Check sheet for the modelled part. Datum: model origin and axes. Units: mm. Coordinates: 2 decimals unless noted, no trailing zeros. Loops run counter-clockwise (first coordinate to the right, second up) from the corner with the lowest first, then second, coordinate; pieces in that order, holes last. Notation, with made-up numbers: (-0.75, -13) - (17.25, -13) arc R13 cw to (17.25, 10) - close; hole circle Ø5 at (-7, 82). An arc over 180 degrees is marked (long way). Use a Markdown table: item, result. Add a question column.
1) Thickness scan on line 1 (X direction, y = 1.8, z = -20); line 2 (Z direction, x = 20, y = 2.65); line 3 (Z direction, x = 29, y = 1.2). Record the ranges inside material, lowest first.
2) Draft check along Z on faces 1 (the cylindrical face through (16.29, 2.465, -17.635)), 2 (the flat face through (0, 2, -51)), 3 (the flat face through (20, 2, 0)), 4 (the flat face through (20, 2, -100)). Enter one of: pulls with the +Z half, pulls with the -Z half, needs draft (parallel to the pull), parting line crosses it, or undercut.
3) Sectioned sample at C-C, the plane x = 20. Enter the section's corners in (y, z), then the cut area to 3 significant figures.
4) Sectioned sample at B-B, the plane z = -20. Enter the section's corners in (x, y).
5) Sectioned sample at D-D, the plane y = 3.55. Enter the section's corners in (x, z), then the cut area to 3 significant figures.
6) Sectioned sample at A-A, the plane x = 36. Enter the section's corners in (y, z).
7) Go/stop test with a flat-tipped pin: P1, Ø1, axis at y = 2.5, z = -11.5, coming from the -X side. Record where the tip stops, or that it passes through.
Autodesk Inventor part; units mm, degrees
ref_plane "YZ Plane" through (0, 0, 0) normal (1, 0, 0) x (0, 1, 0)
ref_plane "XZ Plane" through (0, 0, 0) normal (0, 1, 0) x (-1, 0, 0)
ref_plane "XY Plane" through (0, 0, 0) normal (0, 0, 1) x (1, 0, 0)
sketch "スケッチ1" plane through (0, 0, 0) normal (0, 1, 0) x (-1, 0, 0)
  line L0 (0, 0) -> (-40, 0)
  line L1 (-40, 0) -> (-40, -100)
  line L2 (-40, -100) -> (0, -100)
  line L3 (0, -100) -> (0, 0)
  dimension "d0" = 40
  dimension "d1" = 100
extrude "押し出し1" add sketch "スケッチ1" along normal blind 5
sketch "スケッチ2" plane through (0, 5, 0) normal (0, 1, 0) x (1, 0, 0)
  line L0 (0, 0) -> (40, 0) construction
  line L1 (20, 0) -> (20, 100) construction
  line L2 (40, 100) -> (0, 100) construction
  point P0 (20, 20)
  dimension "d4" = 20
hole "穴1" at (20, 5, -20) direction (0, -1, 0) diameter 8.8 end through all
sketch "スケッチ3" plane through (0, 5, 0) normal (0, 1, 0) x (1, 0, 0)
  circle A0 centre (20, 20) radius 4.4 construction
  circle A1 centre (20, 20) radius 9 construction
  point P0 (0, 0)
  point P1 (11, 20)
  point P2 (20, 11)
  point P3 (29, 20)
  point P4 (20, 29)
  dimension "d12" = 18
  dimension "d15" = 360
hole "穴2" at (11, 5, -20) at (20, 5, -11) at (29, 5, -20) at (20, 5, -29) direction (0, -1, 0) diameter 4.4 end through all
sketch "スケッチ4" plane through (0, 5, 0) normal (0, 1, 0) x (1, 0, 0)
  line L0 (40, 100) -> (0, 100) construction
  line L1 (0, 100) -> (40, 100) construction
  line L2 (40, 100) -> (40, 95) construction
  line L3 (40, 95) -> (0, 95) construction
  line L4 (0, 95) -> (0, 100) construction
  line L5 (0, 100) -> (0, 0)
  line L6 (0, 97.5) -> (40, 97.5) construction
  line L7 (40, 0) -> (40, 100)
  point P0 (4, 97.5)
  point P1 (36, 97.5)
  dimension "d25" = 5
  dimension "d26" = 4
  dimension "d27" = 4
hole "穴3" at (4, 5, -97.5) at (36, 5, -97.5) direction (0, -1, 0) diameter 2.459 end through all
properties part number "shoulder1_sidel_plate"
Solved:
| question | item | result |
|---|---|---|
| 1 | line 1 | x = 0 to 8.8, 13.2 to 15.6, 24.4 to 26.8, 31.2 to 40 |
| 1 | line 2 | z = -100 to -31.2, -26.8 to -24.4, -15.6 to -13.2, -8.8 to 0 |
| 1 | line 3 | z = -100 to -22.2, -17.8 to 0 |
| 2 | face 1 | undercut |
| 2 | face 2 | needs draft |
| 2 | face 3 | pulls with the +Z half |
| 2 | face 4 | pulls with the -Z half |
| 3 | outline | (0, -100) - (5, -100) - (5, -31.2) - (0, -31.2) - close; (0, -26.8) - (5, -26.8) - (5, -24.4) - (0, -24.4) - close; (0, -15.6) - (5, -15.6) - (5, -13.2) - (0, -13.2) - close; (0, -8.8) - (5, -8.8) - (5, 0) - (0, 0) - close |
| 3 | area | 412 mm2 |
| 4 | outline | (0, 0) - (8.8, 0) - (8.8, 5) - (0, 5) - close; (13.2, 0) - (15.6, 0) - (15.6, 5) - (13.2, 5) - close; (24.4, 0) - (26.8, 0) - (26.8, 5) - (24.4, 5) - close; (31.2, 0) - (40, 0) - (40, 5) - (31.2, 5) - close |
| 5 | outline | (0, -100) - (40, -100) - (40, 0) - (0, 0) - close; hole circle Ø2.46 at (4, -97.5); hole circle Ø4.4 at (11, -20); hole circle Ø8.8 at (20, -20); hole circle Ø4.4 at (20, -29); hole circle Ø4.4 at (20, -11); hole circle Ø4.4 at (29, -20); hole circle Ø2.46 at (36, -97.5) |
| 5 | area | 3,870 mm2 |
| 6 | outline | (0, -100) - (5, -100) - (5, -98.73) - (0, -98.73) - close; (0, -96.27) - (5, -96.27) - (5, 0) - (0, 0) - close |
| 7 | P1 | stops at x = 0 |
